The listing builds one solid part. Answer for the finished solid, in the listing's coordinates (mm). A direction names the side the tool comes from. Give positions to 0.01 mm unless a question says otherwise; leave off trailing zeros. Write each loop counter-clockwise with the first axis right and the second up, starting at its lowest first coordinate (ties: lowest second). Pieces come first, ordered by that corner, then holes. Notation, with made-up numbers: M -31,31 L -27,31 A14 ccw -27,35 Z; hole C -11,-24 d5. An arc over 180 degrees is marked long. Return JSON: item names as keys, results as strings.
from build123d import *

# Parameters (mm, degrees)
SKETCH_1_R          = 15
SKETCH_1_R_2        = 1
SKETCH_1_R_3        = 1.5
EXTRUDE_1_DEPTH     = 4
SKETCH_2_R          = 6
SKETCH_2_R_2        = 1.5
EXTRUDE_2_DEPTH     = 1.5
SKETCH_3_R          = 4.5
CUT_EXTRUDE_1_DEPTH = 5


with BuildPart() as part:
    # 草图1 → 凸台-拉伸1 (new body)
    with BuildSketch(Plane(origin=(0, 0, 0), x_dir=(1, 0, 0), z_dir=(0, 1, 0))):
        with Locations(Location((0, 0, 0), (0, 0, 270))):
            Circle(SKETCH_1_R)
        with Locations(Location((0, 12, 0), (0, 0, 270))):
            Circle(SKETCH_1_R_2, mode=Mode.SUBTRACT)
        with Locations(Location((8.485281374, 8.485281374, 0), (0, 0, 270))):
            Circle(SKETCH_1_R_2, mode=Mode.SUBTRACT)
        with Locations(Location((8.485281374, -8.485281374, 0), (0, 0, 90))):
            Circle(SKETCH_1_R_2, mode=Mode.SUBTRACT)
        with Locations(Location((0, -12, 0), (0, 0, 90))):
            Circle(SKETCH_1_R_2, mode=Mode.SUBTRACT)
        with Locations(Location((-8.485281374, -8.485281374, 0), (0, 0, 270))):
            Circle(SKETCH_1_R_2, mode=Mode.SUBTRACT)
        with Locations(Location((-8.485281374, 8.485281374, 0), (0, 0, 90))):
            Circle(SKETCH_1_R_2, mode=Mode.SUBTRACT)
        with Locations(Location((-12, 0, 0), (0, 0, 270))):
            Circle(SKETCH_1_R_2, mode=Mode.SUBTRACT)
        with Locations(Location((12, 0, 0), (0, 0, 90))):
            Circle(SKETCH_1_R_2, mode=Mode.SUBTRACT)
        with Locations(Location((0, 0, 0), (0, 0, 270))):
            Circle(SKETCH_1_R_3, mode=Mode.SUBTRACT)
    extrude(amount=EXTRUDE_1_DEPTH)

    # 草图2 → 凸台-拉伸2 (add)
    with BuildSketch(Plane(origin=(0, 4, 0), x_dir=(1, 0, 0), z_dir=(0, 1, 0))):
        with Locations(Location((0, 0, 0), (0, 0, 270))):
            Circle(SKETCH_2_R)
        with Locations(Location((0, 0, 0), (0, 0, 270))):
            Circle(SKETCH_2_R_2, mode=Mode.SUBTRACT)
    extrude(amount=EXTRUDE_2_DEPTH)

    # 草图3 → 切除-拉伸1 (cut)
    with BuildSketch(Plane.XZ):
        with Locations(Location((0, 0, 0), (0, 0, 270))):
            Circle(SKETCH_3_R)
    extrude(amount=-CUT_EXTRUDE_1_DEPTH, mode=Mode.SUBTRACT)


solid = part.part
Item 1: Determine the mould class of faces 1 (the flat face through (-1.2, 5.5, 1.2)), 2 (the cylindrical face through (-0.6, 2, -12.8)), 3 (the cylindrical face through (0.66, 1.972, -14.985)), 4 (the cylindrical face through (11, 2, 0)) for opening direction X: +X half, -X half, draft (parallel to the pull), parting line (faces both ways), or undercut.
Geometry results:
{"face 1": "draft", "face 2": "undercut", "face 3": "parting line", "face 4": "undercut"}
Item 2: A cutting plane is placed at D-D, the plane z = 12. Write down the section's boundary in (x, y).
Geometry results:
{"outline": "M -9,0 L -1,0 L -1,4 L -9,4 Z; M 1,0 L 9,0 L 9,4 L 1,4 Z"}
Item 3: Given pin 1 Ø3 at (x, z) = (-0.5, -8.5) entering from -Y; pin 2 Ø1.8 at (x, z) = (-12, 0) entering from +Y; pin 3 Ø2.5 at (x, z) = (0, -12) entering from +Y; pin 4 Ø2 at (x, y) = (-2.5, 3) entering from -Z, each flat-ended and moving along its own axis, determine where each tip first touches the part or whether it passes through.
Geometry results:
{"pin 1": "stops at y = 0", "pin 2": "passes through", "pin 3": "stops at y = 4", "pin 4": "stops at z = -14.92"}
Item 4: Which of the six approach directions +Z, -Z, +X, -X, +Y, -Y give full straight-line access (tool end or side, diameter ignored) to faces 5 (the cylindrical face through (-8.529, 1.972, -7.486)), 6 (the flat face through (0.2, 4, 6.5)), 7 (the flat face through (-2, 5, 0))?
Geometry results:
{"face 5": "+Y, -Y", "face 6": "+Y", "face 7": "-Y"}
Item 5: A cutting plane is placed at B-B, the plane z = 0. Write down the section's boundary in (x, y), plus the area to 3 significant figures.
Geometry results:
{"outline": "M -15,0 L -13,0 L -13,4 L -15,4 Z; M -11,0 L -4.5,0 L -4.5,5 L -1.5,5 L -1.5,5.5 L -6,5.5 L -6,4 L -11,4 Z; M 1.5,5 L 4.5,5 L 4.5,0 L 11,0 L 11,4 L 6,4 L 6,5.5 L 1.5,5.5 Z; M 13,0 L 15,0 L 15,4 L 13,4 Z", "area": "75.5 mm2"}
Item 6: Find the intervals of material crossed by line 1 (Z direction, x = -9, y = 3.45); line 2 (X direction, y = 0.75, z = -9.25); line 3 (Y direction, x = -10, z = 4), in increasing order.
Geometry results:
{"line 1": "z = -12 to -9.34, -7.63 to 7.63, 9.34 to 12", "line 2": "x = -11.81 to -9.13, -7.84 to 7.84, 9.13 to 11.81", "line 3": "y = 0 to 4"}
Item 7: A cutting plane is placed at C-C, the plane x = 12. Write down the section's boundary in (y, z), plus the area to 3 significant figures.
Geometry results:
{"outline": "M 0,-9 L 4,-9 L 4,-1 L 0,-1 Z; M 0,1 L 4,1 L 4,9 L 0,9 Z", "area": "64.0 mm2"}
Item 8: A cutting plane is placed at A-A, the plane x = 0. Write down the section's boundary in (y, z), plus the area to 3 significant figures.
Geometry results:
{"outline": "M 0,-15 L 4,-15 L 4,-13 L 0,-13 Z; M 0,-11 L 4,-11 L 4,-6 L 5.5,-6 L 5.5,-1.5 L 5,-1.5 L 5,-4.5 L 0,-4.5 Z; M 0,4.5 L 5,4.5 L 5,1.5 L 5.5,1.5 L 5.5,6 L 4,6 L 4,11 L 0,11 Z; M 0,13 L 4,13 L 4,15 L 0,15 Z", "area": "75.5 mm2"}
